Here's how the part is built. I have some questions about the finished solid (model axes, mm). A direction names the side the tool comes from. Coordinates: 2 decimals unless noted, no trailing zeros. Write each loop counter-clockwise with the first axis right and the second up, starting at its lowest first coordinate (ties: lowest second). Pieces come first, ordered by that corner, then holes. Notation, with made-up numbers: (-29.5, -7) -> (7.5, -7) arc R19 cw to (7.5, 4) -> close; hole circle Ø2 at (-12.5, 18). An arc over 180 degrees is marked (long way). Answer in a Markdown table with one row per item. Add a question column.
from build123d import *

# Parameters (mm, degrees)
F0_W     = 57
F0_H     = 57
F1_DEPTH = 76
F2_R     = 18.05
F2_R_2   = 3.175
F3_DEPTH = 1.6
F4_DEPTH = 21
F5_R     = 2.5
F6_DEPTH = 10


with BuildPart() as f1:
    # F0 (on Top) → F1 (new body)
    with BuildSketch(Plane.XY):
        Rectangle(F0_W, F0_H)
    extrude(amount=F1_DEPTH)

    # F2 (on face) → F3 (join)
    with BuildSketch(Plane.XY.offset(76)):
        Circle(F2_R)
        Circle(F2_R_2, mode=Mode.SUBTRACT)
    extrude(amount=F3_DEPTH)

    # F2 (on face) → F4 (join)
    with BuildSketch(Plane.XY.offset(76)):
        Circle(F2_R_2)
    extrude(amount=F4_DEPTH)

    # F5 (on face) → F6 (cut)
    with BuildSketch(Plane.XY.offset(76)):
        with Locations((-23.5, 23.5)):
            Circle(F5_R)
        with Locations((23.5, 23.5)):
            Circle(F5_R)
        with Locations((23.5, -23.5)):
            Circle(F5_R)
        with Locations((-23.5, -23.5)):
            Circle(F5_R)
    extrude(amount=-F6_DEPTH, mode=Mode.SUBTRACT)


solid = f1.part
Q1. If we mould it in two halves opening along X, with no side actions, what happens to faces 3 (the flat face through (-28.5, 0, 37)), 4 (the cylindrical face through (-25.34, -21.81, 71.07)), 5 (the flat face through (0, 0, 0))? For each: pulls with the +X half, pulls with the -X half, needs draft (parallel to the pull), parting line crosses it, or undercut.
Q2. For faces 1 (the cylindrical face through (-3.91, -17.62, 76.79)), 2 (the flat face through (0, 28.5, 37)), which set-ups out of +Z, -Z, +X, -X, +Y, -Y let a thin tool reach every point of the face, with its end or its side?
Q3. Imagine slicing it at B-B on y = 0. Please give me the cut outline in (x, z) (3 decimals).
Q4. I need wall thicknesses on line 1 (Y direction, x = 23.5, z = 73); line 2 (Y direction, x = 23, z = 68); line 3 (Z direction, x = 5.5, y = 23). Which ranges of each line are inside material? Lowest first, please. Write a range as [from, to].
Q5. I'm going to push flat-ended pins straight in: P1, Ø4, axis at x = -24, y = -22.5, coming from the +Z side; P2, Ø4.5, axis at x = 23.5, y = 23.5, coming from the +Z side. Where does each tip first touch, or does it pass through?
Q6. Imagine slicing it at A-A on z = 70. Please give me the cut outline in (x, y).
Q7. Imagine slicing it at D-D on z = 91.5. Please give me the cut outline in (x, y) (3 decimals), plus the area to 3 significant figures.
Result sheet:
| question | item | result |
|---|---|---|
| 1 | face 3 | pulls with the -X half |
| 1 | face 4 | undercut |
| 1 | face 5 | needs draft |
| 2 | face 1 | +Z |
| 2 | face 2 | +Z, -Z, +X, -X, +Y |
| 3 | outline | (-28.5, 0) -> (28.5, 0) -> (28.5, 76) -> (18.05, 76) -> (18.05, 77.6) -> (3.175, 77.6) -> (3.175, 97) -> (-3.175, 97) -> (-3.175, 77.6) -> (-18.05, 77.6) -> (-18.05, 76) -> (-28.5, 76) -> close |
| 4 | line 1 | y = [-28.5, -26], [-21, 21], [26, 28.5] |
| 4 | line 2 | y = [-28.5, -25.95], [-21.05, 21.05], [25.95, 28.5] |
| 4 | line 3 | z = [0, 76] |
| 5 | P1 | stops at z = 76 |
| 5 | P2 | stops at z = 66 |
| 6 | outline | (-28.5, -28.5) -> (28.5, -28.5) -> (28.5, 28.5) -> (-28.5, 28.5) -> close; hole circle Ø5 at (-23.5, -23.5); hole circle Ø5 at (-23.5, 23.5); hole circle Ø5 at (23.5, -23.5); hole circle Ø5 at (23.5, 23.5) |
| 7 | outline | circle Ø6.35 at (0, 0) |
| 7 | area | 31.7 mm^2 |
